Model file for the job. Use its own axes, mm. Coordinates: 2 decimals unless noted, no trailing zeros. Write each loop counter-clockwise with the first axis right and the second up, starting at its lowest first coordinate (ties: lowest second). Pieces come first, ordered by that corner, then holes. Notation, with made-up numbers: (80.5, 40) - (85.5, 40) arc R17 cw to (85.5, 54) - close; hole circle Ø7 at (23, 44.25). An arc over 180 degrees is marked (long way). Put each result on its own line as item: value. Start each with the question number.
1. Saw through at B-B, the plane y = 28.25. Write the cut outline in (x, z), plus the area to 3 significant figures.
2. Drill centre lines: L1, parallel to Y at x = -7.5, z = -5; L2, parallel to Y at x = -20.5, z = -0.25; L3, parallel to X at y = 30, z = -3.5. Where is each one in solid material? Low to high. Write a range as from..to.
3. Saw through at A-A, the plane z = 2.75. Write the cut outline in (x, y).
4. Saw through at C-C, the plane x = -28.5. Write the cut outline in (y, z).
5. Drop flat-ended pins along their axis: P1, Ø5, axis at y = 31.5, z = 5, coming from the -X side; P2, Ø4, axis at y = 33, z = 3, coming from the +X side; P3, Ø1, axis at y = 32.5, z = 0.5, coming from the -X side. Give the stop position or say it passes through.
```python
from build123d import *

# Parameters (mm, degrees)
EXTRUDE1_DEPTH = 6


with BuildPart() as part:
    # Sketch1 → Extrude1 (new body, symmetric)
    with BuildSketch(Plane.XY):
        with BuildLine():
            Line((-38.224035391, 24.175857425), (-41.98810136, 38.223542865))
            ThreePointArc((-41.98810136, 38.223542865), (-41.470383902, 40.826284287), (-39.090323881, 42))
            Line((-39.090323881, 42), (-7.854139036, 42))
            ThreePointArc((-7.854139036, 42), (-6.609799443, 40.868823297), (-7.617568583, 39.522590361))
            ThreePointArc((-7.617568583, 39.522590361), (-21.825698531, 33.818654373), (-32.875881641, 23.221518175))
            ThreePointArc((-32.875881641, 23.221518175), (-35.853261528, 21.99896609), (-38.224035391, 24.175857425))
        make_face()
    extrude(amount=EXTRUDE1_DEPTH, both=True)


solid = part.part
```
Final values:
1. outline: (-39.32, -6) - (-28.67, -6) - (-28.67, 6) - (-39.32, 6) - close
1. area: 128 mm²
2. L1: y = 39.55..41.95
2. L2: y = 34.64..42
2. L3: x = -39.78..-26.83
3. outline: (-41.99, 38.22) - (-38.22, 24.18) arc R3 ccw to (-32.88, 23.22) arc R40.25 cw to (-7.62, 39.52) arc R1.25 ccw to (-7.85, 42) - (-39.09, 42) arc R3 ccw to start
4. outline: (28.42, -6) - (42, -6) - (42, 6) - (28.42, 6) - close
5. P1: stops at x = -40.86
5. P2: stops at x = -19.88
5. P3: stops at x = -40.59
